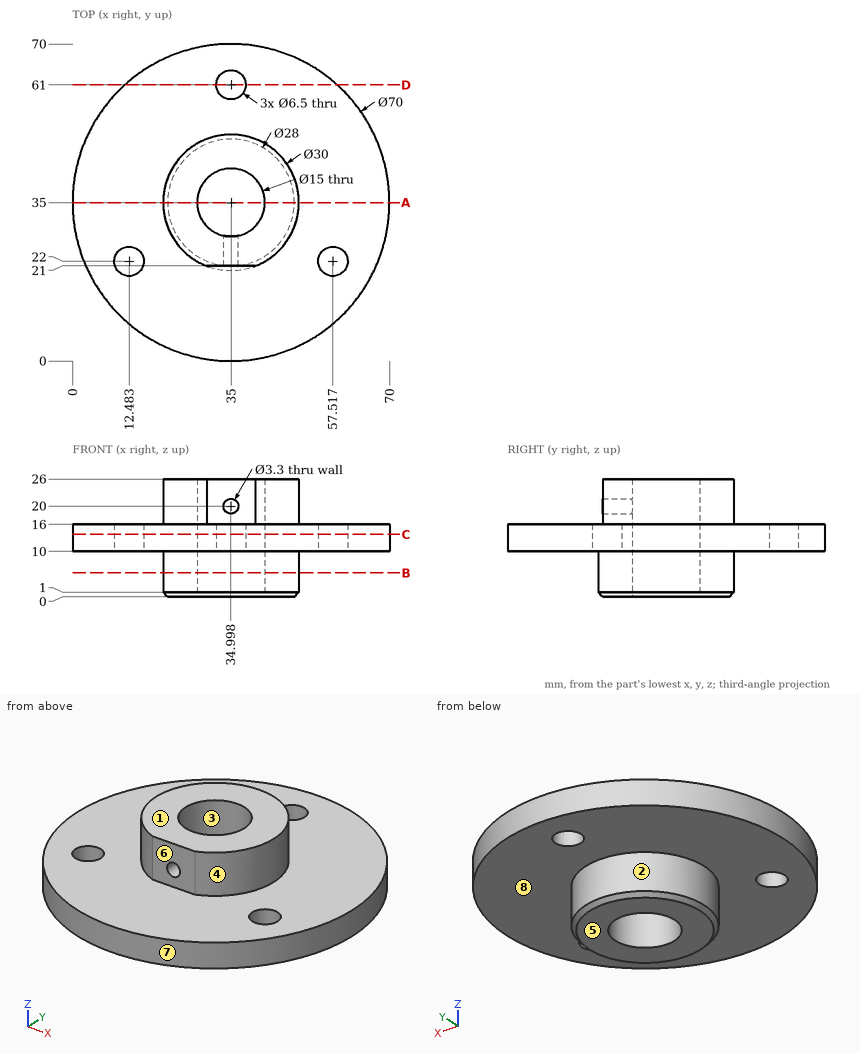
Check sheet for the drawn part. Datum: minimum x, y, z corner. Units: mm. A direction names the side the tool comes from. Coordinates: 2 decimals unless noted, no trailing zeros. Order: outer loops, then holes, each group sorted by start corner. A loop starts at its lowest first (then second) coordinate and runs counter-clockwise, first axis right, second up. Notation, with made-up numbers: (18.5, 80) - (62.5, 80) arc R23 cw to (62.5, 114) - close; hole circle Ø5 at (-19, 22). An arc over 180 degrees is marked (long way). Return JSON: item names as keys, results as strings.
(1) Section check D-D, the plane y = 61. Record the cut outline in (x, z).
Filled sheet:
{"outline": "(11.57, 10) - (31.75, 10) - (31.75, 16) - (11.57, 16) - close; (38.25, 10) - (58.43, 10) - (58.43, 16) - (38.25, 16) - close"}
(2) Section check B-B, the plane z = 5.25. Record the cut outline in (x, y).
Filled sheet:
{"outline": "circle Ø30 at (35, 35); hole circle Ø15 at (35, 35)"}
(3) Section check A-A, the plane y = 35. Record the cut outline in (x, z).
Filled sheet:
{"outline": "(0, 10) - (20, 10) - (20, 1) - (21, 0) - (27.5, 0) - (27.5, 26) - (20, 26) - (20, 16) - (0, 16) - close; (42.5, 0) - (49, 0) - (50, 1) - (50, 10) - (70, 10) - (70, 16) - (50, 16) - (50, 26) - (42.5, 26) - close"}
(4) Access from +Z, -Z, +X, -X, +Y, -Y to the whole of each face (thin tool, end or side, straight path). Record for the marked faces 4, 5, 6, 7 and 8.
Filled sheet:
{"face 4": "+Z", "face 5": "-Z, +X, -X, +Y, -Y", "face 6": "+Z, +X, -X, -Y", "face 7": "+Z, -Z", "face 8": "-Z"}
(5) Mould release check, pull along Y, two halves, no side actions. Record for the marked faces 1, 2 and 3: pulls with the +Y half, pulls with the -Y half, needs draft (parallel to the pull), parting line crosses it, or undercut.
Filled sheet:
{"face 1": "needs draft", "face 2": "parting line crosses it", "face 3": "undercut"}
(6) Thickness scan on line 1 along X through (y, z) = (22, 13.75) (1 decimal); line 2 along Z through (x, y) = (28, 51.5); line 3 along Y through (x, z) = (29.5, 13) (1 decimal). Record the ranges inside material, lowest first.
Filled sheet:
{"line 1": "x = 2.5 to 9.2, 15.7 to 54.3, 60.8 to 67.5", "line 2": "z = 10 to 16", "line 3": "y = 0.4 to 29.9, 40.1 to 69.6"}
(7) Go/stop test with flat-tipped pins: pin 1 (1.5 mm diameter, centred on y = 35, z = 3, fed in from -X); pin 2 (8.5 mm diameter, centred on x = 12.48, y = 22, fed in from -Z); pin 3 (5 mm diameter, centred on x = 32.5, z = 21.5, fed in from -Y); pin 4 (10 mm diameter, centred on y = 57.5, z = 4, fed in from +X). Record where each tip stops, or that it passes through.
Filled sheet:
{"pin 1": "stops at x = 20", "pin 2": "stops at z = 10", "pin 3": "stops at y = 21", "pin 4": "passes through"}
(8) Section check C-C, the plane z = 13.75. Record the cut outline in (x, y), and give its area (3 significant figures).
Filled sheet:
{"outline": "circle Ø70 at (35, 35); hole circle Ø6.5 at (12.48, 22); hole circle Ø15 at (35, 35); hole circle Ø6.5 at (35, 61); hole circle Ø6.5 at (57.52, 22)", "area": "3,570 mm^2"}
